from build123d import *

# Parameters (mm, degrees)
F1_W     = 25.4
F1_H     = 3
F3_R     = 3.0860112986
F4_DEPTH = 48.3815874904


with BuildPart() as f2:
    # F2: sweep along a path in F0
    with BuildLine(Plane.YZ) as f2_path:
        Line((0, 0), (0, 25.4))
        Line((0, 25.4), (25.4, 25.4))
        Line((25.4, 25.4), (25.4, 0))
    # F1 (on Top) → F2 (sweep)
    with BuildSketch(Plane.XY):
        Rectangle(F1_W, F1_H)
    sweep(path=f2_path.line, transition=Transition.RIGHT)

    # F3 (on face) → F4 (cut)
    with BuildSketch(Plane(origin=(0, 26.9, 0), x_dir=(-1, 0, 0), z_dir=(0, 1, 0))):
        with Locations((0, 4.4242767617)):
            Circle(F3_R)
    extrude(amount=-F4_DEPTH, mode=Mode.SUBTRACT)


solid = f2.part
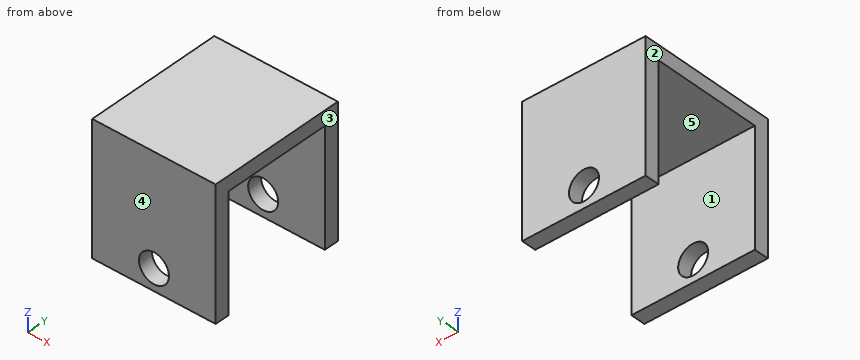
Geometry: final body of the model. Coordinates: model frame, mm. Face numbers are marked on the shaded views. A direction names the side the tool comes from. Round coordinates to 2 decimals unless told otherwise and drop trailing zeros. Loops run counter-clockwise (first coordinate to the right, second up) from the corner with the lowest first, then second, coordinate; pieces in that order, holes last. Notation, with made-up numbers: M 62,-6.5 L 66,-6.5 A29 ccw 66,32.5 Z; hole C 5.25,65.5 d2. An arc over 180 degrees is marked long. Put each result on its own line as item: value. Start each with the question number.
(1) Section query C-C (x = -9.5). Return loops of the section in (y, z).
(2) Material intervals for line 1 along Y through (x, z) = (-8, 22.75); line 2 along Z through (x, y) = (0, 26); line 3 along Z through (x, y) = (1.25, 11.5), sorted ascending. Write a range as [from, to].
(3) Section query A-A (z = 14.5). Return loops of the section in (x, y), then the cut area to 3 significant figures.
(4) Section query B-B (x = 0). Return loops of the section in (y, z).
(5) Section query D-D (y = 25). Return loops of the section in (x, z).
(6) Set-up query: the marked faces 1 and 2. Return all of +Z, -Z, +X, -X, +Y, -Y with unobstructed straight access to the full face (end or side cutting, diameter ignored); none if empty.
(7) Draft query along Y for the marked faces 3, 4 and 5. Return one class per face: +Y half, -Y half, draft (parallel to the pull), parting line (faces both ways), or undercut.
(8) Contact query for flat-ended pins moving along their axis: pin 1 Ø10 at (x, z) = (0, 4.42) entering from -Y; pin 2 Ø12 at (x, y) = (-8, 15) entering from -Z. Output: stop coordinate, or through.
Findings below:
1. outline: M -1.5,0 L 1.5,0 L 1.5,23.9 L 23.9,23.9 L 23.9,0 L 26.9,0 L 26.9,26.9 L -1.5,26.9 Z
2. line 1: y = [-1.5, 1.5], [23.9, 26.9]
2. line 2: z = [0, 1.34], [7.51, 26.9]
2. line 3: z = [23.9, 26.9]
3. outline: M -12.7,-1.5 L 12.7,-1.5 L 12.7,1.5 L -12.7,1.5 Z; M -12.7,23.9 L 12.7,23.9 L 12.7,26.9 L -12.7,26.9 Z
3. area: 152 mm2
4. outline: M -1.5,0 L 1.5,0 L 1.5,1.34 L -1.5,1.34 Z; M -1.5,7.51 L 1.5,7.51 L 1.5,23.9 L 23.9,23.9 L 23.9,7.51 L 26.9,7.51 L 26.9,26.9 L -1.5,26.9 Z; M 23.9,0 L 26.9,0 L 26.9,1.34 L 23.9,1.34 Z
5. outline: M -12.7,0 L 12.7,0 L 12.7,26.9 L -12.7,26.9 Z; hole C 0,4.42 d6.17
6. face 1: -Z, +X, -X
6. face 2: +Z, -Z, -X, +Y, -Y
7. face 3: draft
7. face 4: -Y half
7. face 5: undercut
8. pin 1: stops at y = -1.5
8. pin 2: stops at z = 23.9
